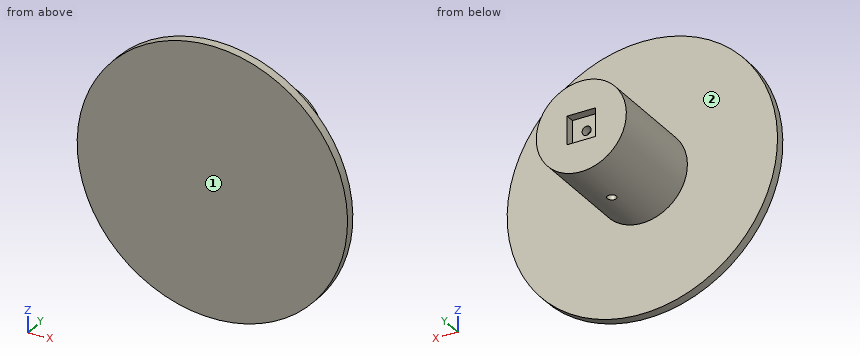
```python
from build123d import *

# Parameters (mm, degrees)
SKETCH_1_R               = 30
EXTRUDE_1_DEPTH          = 2
SKETCH_1_8_R             = 10
EXTRUDE_2_DEPTH          = 25
SKETCH_3_W               = 6.3
SKETCH_3_H               = 6.3
CUT_EXTRUDE_3_DEPTH      = 2
CUT_EXTRUDE_START        = 25
SKETCH_1_9_R             = 1
CUT_EXTRUDE_1_DEPTH      = 4
CUT_EXTRUDE_2_DEPTH      = 50.244289009
CUT_EXTRUDE_2_DEPTH_BACK = 50.244289009
SKETCH_2_R               = 1


with BuildPart() as part:
    # 草图1 → 凸台-拉伸1 (new body)
    with BuildSketch(Plane(origin=(0, 0, 0), x_dir=(1, 0, 0), z_dir=(0, 1, 0))):
        with Locations(Location((0, 0, 0), (0, 0, 270))):
            Circle(SKETCH_1_R)
    extrude(amount=EXTRUDE_1_DEPTH)

    # 草图1<8> → 凸台-拉伸2 (add)
    with BuildSketch(Plane(origin=(0, 0, 0), x_dir=(1, 0, 0), z_dir=(0, 1, 0))):
        with Locations(Location((0, 0, 0), (0, 0, 270))):
            Circle(SKETCH_1_8_R)
    extrude(amount=EXTRUDE_2_DEPTH)

    # 草图3 → 切除-拉伸3 (cut)
    with BuildSketch(Plane(origin=(0, 25, 0), x_dir=(1, 0, 0), z_dir=(0, 1, 0))):
        Rectangle(SKETCH_3_W, SKETCH_3_H)
    extrude(amount=-CUT_EXTRUDE_3_DEPTH, mode=Mode.SUBTRACT)

    # 草图1<9> → 切除-拉伸1 (cut)
    with BuildSketch(Plane(origin=(0, 0, 0), x_dir=(1, 0, 0), z_dir=(0, 1, 0)).offset(CUT_EXTRUDE_START)):
        with Locations(Location((0, 0, 0), (0, 0, 270))):
            Circle(SKETCH_1_9_R)
    extrude(amount=-CUT_EXTRUDE_1_DEPTH, mode=Mode.SUBTRACT)

    # 草图2 → 切除-拉伸2 (cut, two sides: drawn at the far end of the back side and taken through both)
    with BuildSketch(Plane.XY.offset(-CUT_EXTRUDE_2_DEPTH_BACK)):
        with Locations((0, 13.5)):
            Circle(SKETCH_2_R)
    extrude(amount=CUT_EXTRUDE_2_DEPTH + CUT_EXTRUDE_2_DEPTH_BACK, mode=Mode.SUBTRACT)


solid = part.part
```
Check sheet for the modelled part. Datum: model origin and axes. Units: mm. Face numbers are marked on the shaded views. A direction names the side the tool comes from. Coordinates: 2 decimals unless noted, no trailing zeros. Order: outer loops, then holes, each group sorted by start corner. A loop starts at its lowest first (then second) coordinate and runs counter-clockwise, first axis right, second up. Notation, with made-up numbers: M -13,-23.5 L 20,-23.5 A21 ccw 20,14.5 Z; hole C 33,40.25 d4. An arc over 180 degrees is marked long. One line per question, with ' | ' between items. Start each with the question number.
Item 1: Sectioned sample at C-C on y = 13.5. Record the cut outline in (x, z), and give its area (3 significant figures).
Item 2: Access from +Z, -Z, +X, -X, +Y, -Y to the whole of each face (thin tool, end or side, straight path). Record for the marked faces 1 and 2.
Item 3: Material ranges on line 1 (Y direction, x = 0, z = 3.5); line 2 (Y direction, x = 16, z = -9.5); line 3 (X direction, y = 21.8, z = 0), recorded low to high.
Item 4: Sectioned sample at B-B on x = -8.5. Record the cut outline in (y, z).
Item 5: Sectioned sample at D-D on y = 3.25. Record the cut outline in (x, z).
Item 6: Sectioned sample at A-A on z = -2. Record the cut outline in (x, y).
Item 7: Gauge pin test, flat ends, axial feed: P1, Ø2, axis at x = 5.5, y = 7, coming from the -Z side; P2, Ø1.5, axis at x = 17.5, z = 1.5, coming from the +Y side; P3, Ø0.6, axis at y = 23.5, z = -1, coming from the +X side. Record the tip position at first contact, or that the pin passes through.
Answer below:
1) outline: M -1,-9.95 L -1,9.95 A10 ccw Z; M 1,-9.95 A10 ccw 1,9.95 Z | area: 274 mm^2
2) face 1: +Z, -Z, +X, -X, -Y | face 2: +Y
3) line 1: y = 0 to 12.5, 14.5 to 25 | line 2: y = 0 to 2 | line 3: x = -10 to -1, 1 to 10
4) outline: M 0,-28.77 L 2,-28.77 L 2,-5.27 L 25,-5.27 L 25,5.27 L 2,5.27 L 2,28.77 L 0,28.77 Z
5) outline: C 0,0 d20
6) outline: M -29.93,0 L 29.93,0 L 29.93,2 L 9.8,2 L 9.8,25 L 3.15,25 L 3.15,23 L -3.15,23 L -3.15,25 L -9.8,25 L -9.8,2 L -29.93,2 Z; hole C 0,13.5 d2
7) P1: stops at z = -8.93 | P2: stops at y = 2 | P3: stops at x = 9.98
